```python
from build123d import *

# Parameters (mm, degrees)
F1_DEPTH = 12.7
F2_T     = -2
F3_R     = 7
F4_DEPTH = 12.7
F5_R     = 6
F6_DEPTH = 11.43
F7_SIZE  = 3.5


with BuildPart() as f1:
    # F0 (on Top) → F1 (new body)
    with BuildSketch(Plane.XY):
        with BuildLine():
            ThreePointArc((37.637836, 13.542278), (6.25, 10.825318), (-7.090961, 39.366461))
            ThreePointArc((-7.090961, 39.366461), (-20, 34.641016), (-30.546875, 25.824183))
            ThreePointArc((-30.546875, 25.824183), (-12.5, 0), (-30.546875, -25.824183))
            ThreePointArc((-30.546875, -25.824183), (-20, -34.641016), (-7.090961, -39.366461))
            ThreePointArc((-7.090961, -39.366461), (6.25, -10.825318), (37.637836, -13.542278))
            ThreePointArc((37.637836, -13.542278), (40, 0), (37.637836, 13.542278))
        make_face()
    extrude(amount=F1_DEPTH)

    # F2
    f2_openings = [f1.faces().sort_by_distance(p)[0] for p in [
        (0, 0, 12.7),
    ]]
    offset(amount=F2_T, openings=f2_openings)

    # F3 (on face) → F4 (join)
    with BuildSketch(Plane(origin=(0, 0, 0), x_dir=(1, 0, 0), z_dir=(0, 0, -1))):
        Circle(F3_R)
    extrude(amount=-F4_DEPTH)

    # F5 (on face) → F6 (cut)
    with BuildSketch(Plane(origin=(0, 0, 0), x_dir=(1, 0, 0), z_dir=(0, 0, -1))):
        Circle(F5_R)
    extrude(amount=-F6_DEPTH, mode=Mode.SUBTRACT)

    # F7
    f7_edges = [f1.edges().sort_by_distance(p)[0] for p in [
        (40, 0, 0),
        (-20, -34.641016, 0),
        (-20, 34.641016, 0),
    ]]
    chamfer(f7_edges, length=F7_SIZE)


solid = f1.part
```
For this review, take the finished solid that the model builds, in its own axes (mm). A direction names the side the tool comes from. Round coordinates to 2 decimals unless told otherwise and drop trailing zeros. Write each loop counter-clockwise with the first axis right and the second up, starting at its lowest first coordinate (ties: lowest second). Pieces come first, ordered by that corner, then holes. Notation, with made-up numbers: (30, -2) - (58, -2) arc R12 ccw to (58, 2) - close; hole circle Ø9 at (82, 51.5). An arc over 180 degrees is marked (long way). Put each result on its own line as item: value.
Q1. Wall thickness on probe 1 along X at (y, z) = (0.5, 6.75); probe 2 along X at (y, z) = (2.5, 5.5); probe 3 along Y at (x, z) = (0, 4.5): over which ranges is each line inside the solid? List them lowest first.
Solved:
probe 1: x = -12.5 to -10.5, -6.98 to -5.98, 5.98 to 6.98, 38 to 40
probe 2: x = -12.61 to -10.61, -6.54 to -5.45, 5.45 to 6.54, 37.92 to 39.92
probe 3: y = -15.77 to -12.96, -7 to -6, 6 to 7, 12.96 to 15.77
Q2. We need section D-D (y = -18). Give the boundary of the cut face in (x, z).
Solved:
outline: (-19.21, 0) - (-1.89, 0) - (-1.89, 12.7) - (-4.36, 12.7) - (-4.36, 2) - (-16.63, 2) - (-16.63, 12.7) - (-19.21, 12.7) - close
Q3. Mouldability with a two-part tool opening along Y and no side actions: class faces 1 (the face through (40, 0, 8)), 2 (the face through (-20.17, -34.54, 8.04)), 3 (the face through (-3, 7, 0)), 4 (the face through (-19.126, -32.836, 7.275)) as released by +Y, released by -Y, zero draft, split by the parting line, or undercut.
Solved:
face 1: split by the parting line
face 2: released by -Y
face 3: zero draft
face 4: undercut
Q4. Machinability: for faces 5 (the face through (-18.784, 32.901, 1.386)), 6 (the face through (-6, 0, 6)), 7 (the face through (6.466, 2.681, 7.275)), which of the approach directions +Z, -Z, +X, -X, +Y, -Y give a long, thin tool a straight path to every point of the face, cutting with its end or side? Answer none if there is none.
Solved:
face 5: -Z, -X, +Y
face 6: -Z
face 7: +Z
Q5. Insertion check: pin 1 Ø8 at (x, y) = (-10, 24) entering from -Z; pin 2 Ø1.5 at (y, z) = (-13, 10) entering from -X; pin 3 Ø5 at (x, z) = (30.5, 8.5) entering from +Y; pin 4 Ø7 at (x, y) = (0, 0) entering from -Z. Each pin has a flat end and moves straight along its axis. Give the tip position at first contact, or say it passes through.
Solved:
pin 1: stops at z = 0
pin 2: stops at x = -16.18
pin 3: stops at y = 10.41
pin 4: stops at z = 11.43
Q6. We need section B-B (y = 0). Give the boundary of the cut face in (x, z).
Solved:
outline: (-12.5, 0) - (-6, 0) - (-6, 11.43) - (6, 11.43) - (6, 0) - (36.5, 0) - (40, 3.5) - (40, 12.7) - (38, 12.7) - (38, 2) - (7, 2) - (7, 12.7) - (-7, 12.7) - (-7, 2) - (-10.5, 2) - (-10.5, 12.7) - (-12.5, 12.7) - close
Q7. We need section A-A (z = 4.5). Give the boundary of the cut face in (x, y), and give its area (3 significant figures).
Solved:
outline: (-30.55, -25.82) arc R40 ccw to (-7.09, -39.37) arc R27.5 cw to (37.64, -13.54) arc R40 ccw to (37.64, 13.54) arc R27.5 cw to (-7.09, 39.37) arc R40 ccw to (-30.55, 25.82) arc R27.5 cw to start; circle Ø14 at (0, 0); hole (-27.17, -26.56) arc R38 ccw to (-9.42, -36.81) arc R29.5 cw to (36.59, -10.25) arc R38 ccw to (36.59, 10.25) arc R29.5 cw to (-9.42, 36.81) arc R38 ccw to (-27.17, 26.56) arc R29.5 cw to start; hole circle Ø12 at (0, 0)
area: 586 mm2
Q8. We need section C-C (x = 0). Give the boundary of the cut face in (y, z).
Solved:
outline: (-15.77, 0) - (-6, 0) - (-6, 11.43) - (6, 11.43) - (6, 0) - (15.77, 0) - (15.77, 12.7) - (12.96, 12.7) - (12.96, 2) - (7, 2) - (7, 12.7) - (-7, 12.7) - (-7, 2) - (-12.96, 2) - (-12.96, 12.7) - (-15.77, 12.7) - close
